Part model, mm, in its own coordinate system. A direction names the side the tool comes from. Give positions to 0.01 mm unless a question says otherwise; leave off trailing zeros. Order: outer loops, then holes, each group sorted by start corner. A loop starts at its lowest first (then second) coordinate and runs counter-clockwise, first axis right, second up.
from build123d import *

# Parameters (mm, degrees)
BOSS_EXTRUDE1_DEPTH      = 5.08
BOSS_EXTRUDE1_DEPTH_BACK = 19.05
SKETCH1_W                = 69.85
SKETCH1_H                = 18.0655
CUT_EXTRUDE1_DEPTH       = 0.254
CUT_EXTRUDE1_DEPTH_BACK  = 2.254
SKETCH2_W                = 97.536
SKETCH2_H                = 64.008
CUT_EXTRUDE2_DEPTH       = 73.185536469
CUT_EXTRUDE2_DEPTH_BACK  = 73.185536469
SKETCH3_W                = 20.828
SKETCH3_H                = 3.048
CUT_EXTRUDE3_START       = -2.54
SKETCH4_W                = 24.13
SKETCH4_H                = 59.69
CUT_EXTRUDE3_DEPTH       = 2.54
CUT_EXTRUDE4_REACH       = 72.602
SKETCH5_W                = 18.459621809
SKETCH5_H                = 21.336
SKETCH6_W                = 58.928
SKETCH6_H                = 10.9855
CUT_EXTRUDE5_DEPTH       = 15.411621809
SKETCH7_R                = 1.524
CUT_EXTRUDE6_DEPTH       = 73.185536469
CUT_EXTRUDE7_DEPTH       = 2.159
CUT_EXTRUDE9_START       = 59.69
CUT_EXTRUDE9_DEPTH       = 2.159


with BuildPart() as part:
    # Sketch1 → Boss-Extrude1 (new, two sides: drawn at the far end of the back side and taken through both)
    with BuildSketch(Plane(origin=(0, 0, 0), x_dir=(0, 0, -1), z_dir=(1, 0, 0)).offset(-BOSS_EXTRUDE1_DEPTH_BACK)):
        with Locations((31.75, -4.49275)):
            Rectangle(SKETCH1_W, SKETCH1_H)
    extrude(amount=BOSS_EXTRUDE1_DEPTH + BOSS_EXTRUDE1_DEPTH_BACK)

    # Sketch2 → Cut-Extrude1 (cut, two sides: drawn at the far end of the back side and taken through both)
    with BuildSketch(Plane(origin=(0, 2, 0), x_dir=(1, 0, 0), z_dir=(0, 1, 0)).offset(-CUT_EXTRUDE1_DEPTH_BACK)):
        with Locations((-48.26, 31.75)):
            Rectangle(SKETCH2_W, SKETCH2_H)
    extrude(amount=CUT_EXTRUDE1_DEPTH + CUT_EXTRUDE1_DEPTH_BACK, mode=Mode.SUBTRACT)

    # Sketch3 → Cut-Extrude2 (cut, two sides: drawn at the far end of the back side and taken through both)
    with BuildSketch(Plane(origin=(5.08, 0, 0), x_dir=(0, 0, -1), z_dir=(1, 0, 0)).offset(-CUT_EXTRUDE2_DEPTH_BACK)):
        with Locations((29.21, -9.7155)):
            Rectangle(SKETCH3_W, SKETCH3_H)
    extrude(amount=CUT_EXTRUDE2_DEPTH + CUT_EXTRUDE2_DEPTH_BACK, mode=Mode.SUBTRACT)

    # Sketch4 → Cut-Extrude3 (cut)
    with BuildSketch(Plane(origin=(0, 4.54, 0), x_dir=(1, 0, 0), z_dir=(0, 1, 0)).offset(CUT_EXTRUDE3_START)):
        with Locations((-6.985, 31.75)):
            Rectangle(SKETCH4_W, SKETCH4_H)
    extrude(amount=CUT_EXTRUDE3_DEPTH, mode=Mode.SUBTRACT)

    # Cut-Extrude4: up to this face of the body (flat: up to its plane)
    cut_extrude4_end = Plane(part.part.faces().sort_by_distance((-6.985, -11.2395, -29.21))[0])
    # Sketch5 → Cut-Extrude4 (cut, up to the picked face)
    with BuildSketch(Plane(origin=(0, -0.254, 0), x_dir=(1, 0, 0), z_dir=(0, 1, 0)), mode=Mode.PRIVATE) as cut_extrude4_sk1:
        with Locations((-9.820189095, 29.21)):
            Rectangle(SKETCH5_W, SKETCH5_H)
    cut_extrude4_tool1 = split(extrude(cut_extrude4_sk1.sketch, amount=-CUT_EXTRUDE4_REACH, mode=Mode.PRIVATE), bisect_by=cut_extrude4_end, keep=Keep.BOTH, mode=Mode.PRIVATE)
    add(cut_extrude4_tool1.solids().sort_by(Axis((-9.820189, -0.254, -29.21), (0, -1, 0)))[0], mode=Mode.SUBTRACT)

    # Sketch6 → Cut-Extrude5 (cut)
    with BuildSketch(Plane.ZY.offset(19.05)):
        with Locations((-31.75, -5.74675)):
            Rectangle(SKETCH6_W, SKETCH6_H)
    extrude(amount=-CUT_EXTRUDE5_DEPTH, mode=Mode.SUBTRACT)

    # Sketch7 → Cut-Extrude6 (cut, through all)
    with BuildSketch(Plane(origin=(5.08, 0, 0), x_dir=(0, 0, -1), z_dir=(1, 0, 0))):
        with Locations((15.875, -5.9055)):
            Circle(SKETCH7_R)
        with Locations((42.545, -5.9055)):
            Circle(SKETCH7_R)
    extrude(amount=-CUT_EXTRUDE6_DEPTH, mode=Mode.SUBTRACT)

    # Sketch8 → Cut-Extrude7 (cut)
    with BuildSketch(Plane.XY.offset(-61.595)):
        Polygon((-19.05, 2.254), (-2.54, 3.754), (0, 2.254), align=None)
    extrude(amount=-CUT_EXTRUDE7_DEPTH, mode=Mode.SUBTRACT)

    # Sketch8<2> → Cut-Extrude9 (cut)
    with BuildSketch(Plane.XY.offset(-61.595).offset(CUT_EXTRUDE9_START)):
        Polygon((-19.05, 2.254), (-2.54, 3.754), (0, 2.254), align=None)
    extrude(amount=CUT_EXTRUDE9_DEPTH, mode=Mode.SUBTRACT)


solid = part.part
Item 1: Band-saw the part on B-B on z = -26. List the corners of the cut face in (x, y), plus the area to 3 significant figures.
Item 2: Drill centre lines: probe 1 along Z at (x, y) = (-2, 0) (3 decimals); probe 2 along Z at (x, y) = (-1.5, -10.5) (3 decimals); probe 3 along Z at (x, y) = (-2.5, -7) (1 decimal). Where is each one in solid material? Low to high.
Item 3: Drop flat-ended pins along their axis: P1, Ø4, axis at y = -4.5, z = -10.5, coming from the -X side; P2, Ø10, axis at x = -9.5, z = -28.5, coming from the +Y side; P3, Ø1.4, axis at x = 2, z = -32, coming from the +Y side. Give the stop position or say it passes through.
Item 4: Which spindle directions (+Z, -Z, +X, -X, +Y, -Y) get a long thin tool onto all of the face, cutting with end or side? Do faces 4 (the face through (-10, -11.24, -32)), 5 (the face through (-11, -6, -2.286)), 6 (the face through (-10.911, 2.994, -62.659)). Say none if no direction does.
Item 5: Band-saw the part on A-A on y = -10.5. List the corners of the cut face in (x, z) (3 decimals).
Item 6: Band-saw the part on D-D on x = -8. List the corners of the cut face in (y, z) (1 decimal), plus the area to 3 significant figures.
Item 7: Band-saw the part on C-C on z = -5. List the corners of the cut face in (x, y).
Item 8: Pull direction X, two halves, no side cores. Call faces 1 (the face through (-19.05, -12, -32)), 2 (the face through (-7, 4, -1.905)), 3 (the face through (-9, 1, -63.754)): released by +X, released by -X, zero draft, split by the parting line, or undercut.
Working result:
1. outline: (-19.05, -13.53) - (5.08, -13.53) - (5.08, -11.24) - (-19.05, -11.24) - close; (-0.59, -8.19) - (5.08, -8.19) - (5.08, 2) - (0.51, 2) - (0.51, -0.25) - (-0.59, -0.25) - close
1. area: 110 mm2
2. probe 1: z = -66.675 to -63.754, 0.254 to 3.175
2. probe 2: z = -66.675 to -39.878, -18.542 to 3.175
2. probe 3: z = -66.7 to -43.6, -41.5 to -39.9, -18.5 to -16.9, -14.8 to 3.2
3. P1: stops at x = -3.64
3. P2: stops at y = -11.24
3. P3: stops at y = 2
4. face 4: -X
4. face 5: -X, +Y
4. face 6: none
5. outline: (-19.05, -66.675) - (5.08, -66.675) - (5.08, -39.624) - (-0.59, -39.624) - (-0.59, -39.878) - (-3.638, -39.878) - (-3.638, -61.214) - (-19.05, -61.214) - close; (-19.05, -2.286) - (-3.638, -2.286) - (-3.638, -18.542) - (-0.59, -18.542) - (-0.59, -18.796) - (5.08, -18.796) - (5.08, 3.175) - (-19.05, 3.175) - close
6. outline: (-13.5, -66.7) - (4.5, -66.7) - (4.5, -61.6) - (3.3, -61.6) - (3.3, -63.8) - (-0.3, -63.8) - (-0.3, -61.2) - (-11.2, -61.2) - (-11.2, -2.3) - (-0.3, -2.3) - (-0.3, 0.3) - (3.3, 0.3) - (3.3, -1.9) - (4.5, -1.9) - (4.5, 3.2) - (-13.5, 3.2) - close
6. area: 313 mm2
7. outline: (-19.05, -13.53) - (5.08, -13.53) - (5.08, 2) - (0.51, 2) - (0.51, -0.25) - (-3.64, -0.25) - (-3.64, -11.24) - (-19.05, -11.24) - close
8. face 1: released by -X
8. face 2: zero draft
8. face 3: undercut
